The model under review builds one solid part; all positions refer to its coordinate system, in mm. A direction names the side the tool comes from. Give positions to 0.01 mm unless a question says otherwise; leave off trailing zeros. Order: outer loops, then holes, each group sorted by start corner. A loop starts at its lowest first (then second) coordinate and runs counter-clockwise, first axis right, second up.
```python
from build123d import *

# Parameters (mm, degrees)
SKETCH1_W           = 43.57
SKETCH1_H           = 63.5
BOSS_EXTRUDE1_DEPTH = 55
CUT_EXTRUDE2_DEPTH  = 95.634004988
SKETCH4_W           = 43.57
SKETCH4_H           = 55
SKETCH4_W_2         = 6
SKETCH4_H_2         = 15
BOSS_EXTRUDE2_DEPTH = 9
SKETCH5_R           = 1
CUT_EXTRUDE3_DEPTH  = 1
BOSS_EXTRUDE3_START = -26.785
BOSS_EXTRUDE3_DEPTH = 10
SKETCH7_R           = 2
CUT_EXTRUDE4_DEPTH  = 2
SKETCH13_W          = 9
SKETCH13_H          = 8
BOSS_EXTRUDE6_DEPTH = 10
FILLET12_R          = 3
FILLET2_R           = 1
BOSS_EXTRUDE4_DEPTH = 10
BOSS_EXTRUDE5_DEPTH = 7.5
CUT_EXTRUDE11_DEPTH = 174.835946297
LPATTERN1_COUNT     = 5
LPATTERN1_PITCH     = 12
FILLET9_R           = 1
FILLET11_R          = 11
SKETCH14_R          = 2
CUT_EXTRUDE12_DEPTH = 156.361674811
SKETCH15_W          = 15
SKETCH15_H          = 33
CUT_EXTRUDE13_DEPTH = 33
SKETCH16_W          = 15
SKETCH16_H          = 25
CUT_EXTRUDE14_DEPTH = 26
SKETCH18_R          = 0.8
CUT_EXTRUDE15_DEPTH = 8
SKETCH19_W          = 15
SKETCH19_H          = 5
CUT_EXTRUDE16_DEPTH = 25
SKETCH20_W          = 38.57
SKETCH20_H          = 51
CUT_EXTRUDE17_DEPTH = 33
SKETCH21_W          = 4
SKETCH21_H          = 13
CUT_EXTRUDE18_DEPTH = 27


with BuildPart() as part:
    # Sketch1 → Boss-Extrude1 (new body)
    with BuildSketch(Plane.XY):
        with Locations((21.785, 31.75)):
            Rectangle(SKETCH1_W, SKETCH1_H)
    extrude(amount=BOSS_EXTRUDE1_DEPTH)

    # Sketch3 → Cut-Extrude2 (cut, through all)
    with BuildSketch(Plane(origin=(43.57, 0, 0), x_dir=(0, 0, -1), z_dir=(1, 0, 0))):
        with BuildLine():
            Line((-29.5, 0), (-29.5, 1.5))
            ThreePointArc((-29.5, 1.5), (-29.060660172, 2.560660172), (-28, 3))
            Line((-28, 3), (-27, 3))
            ThreePointArc((-27, 3), (-25.939339828, 2.560660172), (-25.5, 1.5))
            Line((-25.5, 1.5), (-25.5, 0))
            Line((-25.5, 0), (-22.5, 0))
            Line((-22.5, 0), (-22.5, 3.5))
            ThreePointArc((-22.5, 3.5), (-22.939339828, 4.560660172), (-24, 5))
            Line((-24, 5), (-31, 5))
            ThreePointArc((-31, 5), (-32.060660172, 4.560660172), (-32.5, 3.5))
            Line((-32.5, 3.5), (-32.5, 0))
            Line((-32.5, 0), (-29.5, 0))
        make_face()
    extrude(amount=-CUT_EXTRUDE2_DEPTH, mode=Mode.SUBTRACT)


with BuildPart() as cut_extrude2_piece_1:
    # of the separate pieces the step leaves, piece 1, a body of its own (cut_extrude2_pieces)
    add(part.part.solids().sort_by_distance((0, 0, 0))[0])



with BuildPart() as cut_extrude2_piece_2:
    # of the separate pieces the step leaves, piece 2, a body of its own (cut_extrude2_pieces)
    add(part.part.solids().sort_by_distance((43.57, 0, 25.5))[0])


with BuildPart() as cut_extrude2_piece_1_1:
    add(cut_extrude2_piece_1.part)

    add(cut_extrude2_piece_2.part)  # Boss-Extrude2 merges Cut-Extrude2 piece 2
    # Sketch4 → Boss-Extrude2 (add)
    with BuildSketch(Plane.XZ):
        with Locations((21.785, 27.5)):
            Rectangle(SKETCH4_W, SKETCH4_H)
        with Locations((10.785, 27.5)):
            Rectangle(SKETCH4_W_2, SKETCH4_H_2, mode=Mode.SUBTRACT)
        with Locations((32.785, 27.5)):
            Rectangle(SKETCH4_W_2, SKETCH4_H_2, mode=Mode.SUBTRACT)
    extrude(amount=-BOSS_EXTRUDE2_DEPTH)

    # Sketch5 → Cut-Extrude3 (cut)
    with BuildSketch(Plane(origin=(0, 0, 0), x_dir=(-1, 0, 0), z_dir=(0, -1, 0))):
        with Locations(Location((-21.785, -27.5, 0), (0, 0, 90))):
            Circle(SKETCH5_R)
    extrude(amount=-CUT_EXTRUDE3_DEPTH, mode=Mode.SUBTRACT)

    # Sketch6 → Boss-Extrude3 (add)
    with BuildSketch(Plane.ZY.offset(BOSS_EXTRUDE3_START)):
        with BuildLine():
            Line((55, 48.5), (75, 48.5))
            ThreePointArc((75, 48.5), (80, 53.5), (75, 58.5))
            Line((75, 58.5), (55, 58.5))
            ThreePointArc((55, 58.5), (50, 53.5), (55, 48.5))
        make_face()
    boss_extrude3 = extrude(amount=BOSS_EXTRUDE3_DEPTH)

    # Mirror1: Boss-Extrude3 across plane
    add(boss_extrude3.mirror(Plane(origin=(0, 0, 27.5), x_dir=(1, 0, 0), z_dir=(0, 0, -1))))

    # Sketch7 → Cut-Extrude4 (cut, symmetric)
    # profile 1 of 3: a face of its own
    with BuildSketch(Plane.ZY.offset(-21.785)):
        with BuildLine():
            ThreePointArc((75, 58.5), (71.464466094, 57.035533906), (70, 53.5))
            ThreePointArc((70, 53.5), (71.464466094, 49.964466094), (75, 48.5))
            ThreePointArc((75, 48.5), (78.535533906, 49.964466094), (80, 53.5))
            ThreePointArc((80, 53.5), (78.535533906, 57.035533906), (75, 58.5))
        make_face()
        with Locations(Location((75, 53.5, 0), (0, 0, 270))):
            Circle(SKETCH7_R, mode=Mode.SUBTRACT)
    # profile 2 of 3: a face of its own
    with BuildSketch(Plane.ZY.offset(-21.785)):
        with BuildLine():
            Line((70, 58.5), (70, 53.5))
            ThreePointArc((70, 53.5), (71.464466094, 57.035533906), (75, 58.5))
            Line((75, 58.5), (70, 58.5))
        make_face()
    # profile 3 of 3: a face of its own
    with BuildSketch(Plane.ZY.offset(-21.785)):
        with BuildLine():
            ThreePointArc((75, 48.5), (71.464466094, 49.964466094), (70, 53.5))
            Line((70, 53.5), (70, 48.5))
            Line((70, 48.5), (75, 48.5))
        make_face()
    extrude(amount=CUT_EXTRUDE4_DEPTH, both=True, mode=Mode.SUBTRACT)

    # Sketch13 → Boss-Extrude6 (add)
    with BuildSketch(Plane(origin=(26.785, 0, 0), x_dir=(0, 0, -1), z_dir=(1, 0, 0))):
        with Locations((-65.5, 62.5)):
            Rectangle(SKETCH13_W, SKETCH13_H)
    extrude(amount=-BOSS_EXTRUDE6_DEPTH)

    # Fillet12
    fillet12_edges = [cut_extrude2_piece_1_1.edges().sort_by_distance(p)[0] for p in [
        (21.785, 66.5, 61),
        (21.785, 66.5, 70),
        (21.785, 58.5, 61),
    ]]
    fillet(fillet12_edges, radius=FILLET12_R)

    # Fillet2
    fillet2_edges = [cut_extrude2_piece_1_1.edges().sort_by_distance(p)[0] for p in [
        (16.785, 48.5, 65),
        (16.785, 53.5, 80),
        (16.785, 58.5, 72.5),
        (26.785, 48.5, 65),
        (26.785, 53.5, 80),
        (26.785, 58.5, 72.5),
    ]]
    fillet(fillet2_edges, radius=FILLET2_R)

    # Sketch10 → Boss-Extrude4 (add)
    with BuildSketch(Plane.ZY.offset(-16.785)):
        with BuildLine():
            Line((-25, 53.5), (-25, 78.5))
            Line((-25, 78.5), (-17.5, 78.5))
            Line((-17.5, 78.5), (-17.5, 58.5))
            Line((-17.5, 58.5), (-20, 58.5))
            ThreePointArc((-20, 58.5), (-23.535533906, 57.035533906), (-25, 53.5))
        make_face()
    extrude(amount=-BOSS_EXTRUDE4_DEPTH)

    # Sketch11 → Boss-Extrude5 (add)
    with BuildSketch(Plane(origin=(0, 0, -25), x_dir=(-1, 0, 0), z_dir=(0, 0, -1))):
        Polygon((-21.785, 63.5), (8.215, 78.5), (8.215, 128.5), (-51.785, 128.5), (-51.785, 78.5), align=None)
    extrude(amount=-BOSS_EXTRUDE5_DEPTH)

    # Sketch12 → Cut-Extrude11 (cut, through all)
    with BuildSketch(Plane(origin=(0, 0, -25), x_dir=(-1, 0, 0), z_dir=(0, 0, -1))):
        Polygon((-51.785, 128.5), (-45.785, 122.5), (-39.785, 128.5), align=None)
    cut_extrude11 = extrude(amount=-CUT_EXTRUDE11_DEPTH, mode=Mode.SUBTRACT)

    # LPattern1: Cut-Extrude11 ×5
    with Locations(*[(-i * LPATTERN1_PITCH, 0, 0) for i in range(1, LPATTERN1_COUNT)]):
        add(cut_extrude11, mode=Mode.SUBTRACT)

    # Fillet9
    fillet9_edges = [cut_extrude2_piece_1_1.edges().sort_by_distance(p)[0] for p in [
        (-8.215, 128.5, -21.25),
        (51.785, 128.5, -21.25),
    ]]
    fillet(fillet9_edges, radius=FILLET9_R)

    # Fillet11
    fillet11_edges = [cut_extrude2_piece_1_1.edges().sort_by_distance(p)[0] for p in [
        (-8.215, 78.5, -21.25),
        (51.785, 78.5, -21.25),
    ]]
    fillet(fillet11_edges, radius=FILLET11_R)

    # Sketch14 → Cut-Extrude12 (cut, through all)
    with BuildSketch(Plane.ZY.offset(-16.785)):
        with Locations(Location((65.5, 63, 0), (0, 0, 270))):
            Circle(SKETCH14_R)
    extrude(amount=-CUT_EXTRUDE12_DEPTH, mode=Mode.SUBTRACT)

    # Sketch15 → Cut-Extrude13 (cut)
    with BuildSketch(Plane(origin=(0, 63.5, 0), x_dir=(1, 0, 0), z_dir=(0, 1, 0))):
        with Locations((21.785, -27.5)):
            Rectangle(SKETCH15_W, SKETCH15_H)
    extrude(amount=-CUT_EXTRUDE13_DEPTH, mode=Mode.SUBTRACT)

    # Sketch16 → Cut-Extrude14 (cut)
    with BuildSketch(Plane(origin=(0, 30.5, 0), x_dir=(1, 0, 0), z_dir=(0, 1, 0))):
        with Locations((21.785, -27.5)):
            Rectangle(SKETCH16_W, SKETCH16_H)
    extrude(amount=-CUT_EXTRUDE14_DEPTH, mode=Mode.SUBTRACT)

    # Sketch18 → Cut-Extrude15 (cut)
    with BuildSketch(Plane(origin=(0, 30.5, 0), x_dir=(1, 0, 0), z_dir=(0, 1, 0))):
        with Locations(Location((21.785, -13.6, 0), (0, 0, 270))):
            Circle(SKETCH18_R)
        with Locations(Location((21.785, -41.4, 0), (0, 0, 270))):
            Circle(SKETCH18_R)
    extrude(amount=-CUT_EXTRUDE15_DEPTH, mode=Mode.SUBTRACT)

    # Sketch19 → Cut-Extrude16 (cut)
    with BuildSketch(Plane(origin=(0, 4.5, 0), x_dir=(1, 0, 0), z_dir=(0, 1, 0))):
        with Locations((21.785, -17.5)):
            Rectangle(SKETCH19_W, SKETCH19_H)
    extrude(amount=-CUT_EXTRUDE16_DEPTH, mode=Mode.SUBTRACT)

    # Sketch20 → Cut-Extrude17 (cut)
    with BuildSketch(Plane(origin=(0, 63.5, 0), x_dir=(1, 0, 0), z_dir=(0, 1, 0))):
        with Locations((21.785, -27.5)):
            Rectangle(SKETCH20_W, SKETCH20_H)
    extrude(amount=-CUT_EXTRUDE17_DEPTH, mode=Mode.SUBTRACT)

    # Sketch21 → Cut-Extrude18 (cut)
    with BuildSketch(Plane.XY.offset(70)):
        with Locations((21.785, 52)):
            Rectangle(SKETCH21_W, SKETCH21_H)
    extrude(amount=-CUT_EXTRUDE18_DEPTH, mode=Mode.SUBTRACT)


solid = cut_extrude2_piece_1_1.part
```
Item 1: Take a section at D-D (y = 9). Give the boundary of the cut face in (x, z) (3 decimals).
Values found:
outline: (0, 0) - (43.57, 0) - (43.57, 55) - (0, 55) - close; hole (14.285, 15) - (29.285, 15) - (29.285, 40) - (14.285, 40) - close
Item 2: Draft analysis for pull direction X (two halves, no side actions). For faces 1 (the flat face through (11, 2, 22.5)), 2 (the flat face through (36.827, 125.542, -21.303)), 3 (the flat face through (26.785, 55, -15)), 4 (the cylindrical face through (21.86, 49.93, -23.5)), state which applies: released by +X, released by -X, zero draft, split by the parting line, or undercut.
Values found:
face 1: undercut
face 2: undercut
face 3: released by +X
face 4: zero draft
Item 3: Take a section at C-C (z = 50). Give the boundary of the cut face in (x, y).
Values found:
outline: (0, 0) - (43.57, 0) - (43.57, 63.5) - (41.07, 63.5) - (41.07, 30.5) - (2.5, 30.5) - (2.5, 63.5) - (0, 63.5) - close
Item 4: For faces 5 (the cylindrical face through (21.72, 65.6, 61.86)), 6 (the flat face through (-4.331, 124.616, -21.303)), 7 (the flat face through (30, 30.5, 27)), 8 (the flat face through (16.785, 55, -15)), list the 3-axis set-ups (+Z, -Z, +X, -X, +Y, -Y) from which the entire face can be reached by the end or side of a thin tool; tool diameter is ignored.
Values found:
face 5: +X, -X, +Y
face 6: +Z, -Z, +Y
face 7: +Y
face 8: -Z, -X, -Y
Item 5: Take a section at B-B (y = 34). Give the boundary of the cut face in (x, z), and give its area (3 significant figures).
Values found:
outline: (0, 0) - (43.57, 0) - (43.57, 55) - (0, 55) - close; hole (2.5, 2) - (41.07, 2) - (41.07, 53) - (2.5, 53) - close
area: 429 mm2
Item 6: Clearance check with flat-ended pins moving along their axes: pin 1 Ø12 at (x, y) = (21, 15.5) entering from -Z; pin 2 Ø3.5 at (x, z) = (18.5, 56) entering from +Y; pin 3 Ø0.6 at (x, z) = (18.5, 67) entering from -Y. State where each tip first meets the part, or that it passes through.
Values found:
pin 1: stops at z = 0
pin 2: stops at y = 63.5
pin 3: stops at y = 48.5
Item 7: Take a section at A-A (z = 65.5). Give the boundary of the cut face in (x, y) (3 decimals).
Values found:
outline: (16.785, 49.5) arc R1 ccw to (17.785, 48.5) - (19.785, 48.5) - (19.785, 58.5) - (23.785, 58.5) - (23.785, 48.5) - (25.785, 48.5) arc R1 ccw to (26.785, 49.5) - (26.785, 61) - (16.785, 61) - close; (16.785, 65) - (26.785, 65) - (26.785, 66.5) - (16.785, 66.5) - close
Item 8: For line 1 (X direction, y = 0.6, z = 27.5) (3 decimals); line 2 (X direction, y = 8, z = 26) (3 decimals); line 3 (Z direction, x = 24, y = 22.5), list the stretches that pass through material, from the lowest coordinate up.
Values found:
line 1: x = 0 to 20.785, 22.785 to 43.57
line 2: x = 0 to 14.285, 29.285 to 43.57
line 3: z = 0 to 15, 40 to 55
